Model file for the job. Use its own axes, mm. A direction names the side the tool comes from. Give positions to 0.01 mm unless a question says otherwise; leave off trailing zeros. Write each loop counter-clockwise with the first axis right and the second up, starting at its lowest first coordinate (ties: lowest second). Pieces come first, ordered by that corner, then holes. Notation, with made-up numbers: (35, 17) - (44, 17) arc R27 cw to (44, 41) - close; hole circle Ø3 at (-31, -31.75). An arc over 180 degrees is marked (long way). Use CSV: the item, a comma, the result in double quotes.
from build123d import *

# Parameters (mm, degrees)
EXTRUDE1_DEPTH    = 230
SKETCH2_R         = 50
EXTRUDE4_DEPTH    = 20
SKETCH5_R         = 175
EXTRUDE5_DEPTH    = 20
SKETCH6_R         = 50
EXTRUDE6_DEPTH    = 90
CHAMFER2_SIZE     = 40
CHAMFER2_SIZE2    = 12
SKETCH7_R         = 80
EXTRUDE7_DEPTH    = 30
SKETCH8_R         = 12
EXTRUDE8_DEPTH    = 50
CIRPATTERN1_COUNT = 10


with BuildPart() as part:
    # Sketch1 → Extrude1 (new body)
    with BuildSketch(Plane.XY):
        with BuildLine():
            Line((10, 0), (90, 0))
            ThreePointArc((90, 0), (97.071067812, 2.928932188), (100, 10))
            Line((100, 10), (100, 90))
            ThreePointArc((100, 90), (97.071067812, 97.071067812), (90, 100))
            Line((90, 100), (10, 100))
            ThreePointArc((10, 100), (2.928932188, 97.071067812), (0, 90))
            Line((0, 90), (0, 10))
            ThreePointArc((0, 10), (2.928932188, 2.928932188), (10, 0))
        make_face()
    extrude(amount=EXTRUDE1_DEPTH)

    # Sketch2 → Extrude4 (add)
    with BuildSketch(Plane.XY.offset(230)):
        with Locations((50, 50)):
            Circle(SKETCH2_R)
    extrude(amount=EXTRUDE4_DEPTH)

    # Sketch5 → Extrude5 (add)
    with BuildSketch(Plane.XY.offset(250)):
        with Locations((50, 50)):
            Circle(SKETCH5_R)
    extrude(amount=EXTRUDE5_DEPTH)

    # Sketch6 → Extrude6 (add)
    with BuildSketch(Plane.XY.offset(270)):
        with Locations((50, 50)):
            Circle(SKETCH6_R)
    extrude(amount=EXTRUDE6_DEPTH)

    # Chamfer2
    chamfer2_edges = [part.edges().sort_by_distance(p)[0] for p in [
        (0, 50, 360),
    ]]
    chamfer2_side = [part.faces().sort_by_distance(p)[0] for p in [
        (0, 50, 315),
    ]]
    chamfer(chamfer2_edges, length=CHAMFER2_SIZE, length2=CHAMFER2_SIZE2, reference=chamfer2_side[0])

    # Sketch7 → Extrude7 (add)
    with BuildSketch(Plane.XY.offset(270)):
        with Locations((50, 50)):
            Circle(SKETCH7_R)
    extrude(amount=EXTRUDE7_DEPTH)

    # Sketch8 → Extrude8 (add)
    with BuildSketch(Plane.XY.offset(270)):
        with Locations((-90, 50)):
            Circle(SKETCH8_R)
    extrude8 = extrude(amount=EXTRUDE8_DEPTH)

    # CirPattern1: Extrude8 ×10 about axis
    cirpattern1_axis = Axis((50, 50, 0), (0, 0, 1))
    for i in range(1, CIRPATTERN1_COUNT):
        add(extrude8.rotate(cirpattern1_axis, i * 360 / CIRPATTERN1_COUNT))


solid = part.part
(1) Saw through at C-C, the plane y = -83. List the corners of the cut face in (x, z).
Checked values:
outline,"(-63.74, 250) - (163.74, 250) - (163.74, 270) - (105.26, 270) - (105.26, 320) - (81.26, 320) - (81.26, 270) - (18.74, 270) - (18.74, 320) - (-5.26, 320) - (-5.26, 270) - (-63.74, 270) - close"
(2) 3-axis set-ups, long thin cutter, end or side, ignore diameter. For faces 1 (the face through (10.74, -94.46, 294.65)), 2 (the face through (190, 50, 320)), 3 (the face through (12, 90, 230)): which of +Z, -Z, +X, -X, +Y, -Y reach the whole face in a straight line?
Checked values:
face 1,"+Z"
face 2,"+Z, +X, +Y, -Y"
face 3,"-X, +Y"
(3) Flat gauge pins, fed straight in: P1, Ø19, axis at x = -91, y = 53.5, coming from the +Z side; P2, Ø1, axis at x = 22, y = 155.5, coming from the -Z side; P3, Ø24, axis at x = 61, z = 102.5, coming from the -Y side. Where does each tip first touch, or does it go through?
Checked values:
P1,"stops at z = 320"
P2,"stops at z = 250"
P3,"stops at y = 0"
(4) Saw through at D-D, the plane y = 157. List the corners of the cut face in (x, z).
Checked values:
outline,"(-88.48, 250) - (188.48, 250) - (188.48, 270) - (-88.48, 270) - close"
(5) Saw through at A-A, the plane x = -90. List the corners of the cut face in (y, z), then the cut area to 3 significant figures.
Checked values:
outline,"(-55, 250) - (155, 250) - (155, 270) - (62, 270) - (62, 320) - (38, 320) - (38, 270) - (-55, 270) - close"
area,"5,400 mm^2"
(6) Wall check: probe 1 along Y at (x, z) = (96, 308); probe 2 along Y at (x, z) = (43, 136.5); probe 3 along Z at (x, y) = (24, 112). Give the ranges that are in metal, low to high. Write a range as [from, to].
Checked values:
probe 1,"y = [-94.83, -71.46], [30.4, 69.6], [171.46, 194.83]"
probe 2,"y = [0, 100]"
probe 3,"z = [250, 300]"
(7) Saw through at B-B, the plane z = 121.5. List the corners of the cut face in (x, y), then the cut area to 3 significant figures.
Checked values:
outline,"(0, 10) arc R10 ccw to (10, 0) - (90, 0) arc R10 ccw to (100, 10) - (100, 90) arc R10 ccw to (90, 100) - (10, 100) arc R10 ccw to (0, 90) - close"
area,"9,910 mm^2"
(8) Pull direction X, two halves, no side cores. Call faces 4 (the face through (-90, 50, 320)), 5 (the face through (86.872, 34.712, 353.613)), 6 (the face through (-101.99, 50.53, 294.65)), 7 (the face through (3.01, 97.15, 113.39)): released by +X, released by -X, zero draft, split by the parting line, or undercut.
Checked values:
face 4,"zero draft"
face 5,"split by the parting line"
face 6,"undercut"
face 7,"released by -X"
